```python
from build123d import *

# Parameters (mm, degrees)
F1_DEPTH = 600
F2_W     = 200
F2_H     = 260
F3_DEPTH = 250.001
F4_R     = 110
F5_DEPTH = 250


with BuildPart() as f1:
    # F0 (on Front) → F1 (new body)
    with BuildSketch(Plane.XZ):
        with BuildLine():
            Line((600, 125), (-600, 125))
            Line((-600, 125), (-600, -125))
            Line((-600, -125), (-180, -125))
            ThreePointArc((-180, -125), (0, 55), (180, -125))
            Line((180, -125), (600, -125))
            Line((600, -125), (600, 125))
        make_face()
    extrude(amount=F1_DEPTH)

    # F2 (on face) → F3 (cut, through all)
    with BuildSketch(Plane.XY.offset(125)):
        with Locations((-500, -300)):
            Rectangle(F2_W, F2_H)
        with Locations((500, -300)):
            Rectangle(F2_W, F2_H)
    extrude(amount=-F3_DEPTH, mode=Mode.SUBTRACT)

    # F4 (on face) → F5 (join)
    with BuildSketch(Plane.XY.offset(125)):
        Polygon((300, -300), (0, 0), (-300, -300), (0, -600), align=None)
        with Locations((0, -300)):
            Circle(F4_R, mode=Mode.SUBTRACT)
    extrude(amount=F5_DEPTH)


solid = f1.part
```
Check sheet for the modelled part. Datum: model origin and axes. Units: mm. A direction names the side the tool comes from. Round coordinates to 2 decimals unless told otherwise and drop trailing zeros. Order: outer loops, then holes, each group sorted by start corner. A loop starts at its lowest first (then second) coordinate and runs counter-clockwise, first axis right, second up. Notation, with made-up numbers: (-5, 53) -> (52, 53) arc R8 ccw to (52, 60) -> close; hole circle Ø9 at (-23, 77.5). An arc over 180 degrees is marked (long way). One line per item, written item: value. Start each with the question number.
Q1. Mould release check, pull along Y, two halves, no side actions. Record for faces 1 (the face through (-8, -600, 57)), 2 (the face through (-346, -296, -125)), 3 (the face through (-14.32, -190.936, 248.25)): pulls with the +Y half, pulls with the -Y half, needs draft (parallel to the pull), parting line crosses it, or undercut.
Q2. Cross-section at B-B (z = 30). Record the boundary of the cut face in (x, y).
Q3. Set-up check for faces 4 (the face through (-152, -448, 248)), 5 (the face through (-400, -302, 2)), 6 (the face through (-148, -148, 248)), 7 (the face through (-362, -296, 125)): record each of +Z, -Z, +X, -X, +Y, -Y from which the full face is reachable in a straight line by a thin tool's end or side.
Q4. Gauge pin test, flat ends, axial feed: pin 1 Ø4 at (y, z) = (-192.5, 254.5) entering from -X; pin 2 Ø8 at (y, z) = (-398.5, 71.5) entering from +X; pin 3 Ø8 at (y, z) = (-125.5, 176) entering from -X. Record the tip position at first contact, or that the pin passes through.
Q5. Thickness scan on line 1 (Y direction, x = -445, z = 11); line 2 (Y direction, x = 0, z = 237.5); line 3 (Z direction, x = 272.5, y = -474). Record the ranges inside material, lowest first.
Q6. Cross-section at A-A (x = -418.5). Record the boundary of the cut face in (y, z).
Q7. Cross-section at C-C (x = 226). Record the boundary of the cut face in (y, z).
Q8. Cross-section at D-D (y = -105.5). Record the boundary of the cut face in (x, z).
Completed:
1. face 1: pulls with the -Y half
1. face 2: needs draft
1. face 3: undercut
2. outline: (-600, -600) -> (-91.52, -600) -> (-91.52, 0) -> (-600, 0) -> (-600, -170) -> (-400, -170) -> (-400, -430) -> (-600, -430) -> close; (91.52, -600) -> (600, -600) -> (600, -430) -> (400, -430) -> (400, -170) -> (600, -170) -> (600, 0) -> (91.52, 0) -> close
3. face 4: +Z, -X, -Y
3. face 5: +Z, -Z, -X
3. face 6: +Z, -X, +Y
3. face 7: +Z, -X
4. pin 1: stops at x = -194.5
4. pin 2: stops at x = 400
4. pin 3: stops at x = -129.5
5. line 1: y = -600 to -430, -170 to 0
5. line 2: y = -600 to -410, -190 to 0
5. line 3: z = -125 to 125
6. outline: (-600, -125) -> (-430, -125) -> (-430, 125) -> (-600, 125) -> close; (-170, -125) -> (0, -125) -> (0, 125) -> (-170, 125) -> close
7. outline: (-600, -125) -> (0, -125) -> (0, 125) -> (-226, 125) -> (-226, 375) -> (-374, 375) -> (-374, 125) -> (-600, 125) -> close
8. outline: (-600, -125) -> (-180, -125) arc R180 cw to (180, -125) -> (600, -125) -> (600, 125) -> (105.5, 125) -> (105.5, 375) -> (-105.5, 375) -> (-105.5, 125) -> (-600, 125) -> close
